Geometry: final body of the model. Coordinates: model frame, mm. A direction names the side the tool comes from. Round coordinates to 2 decimals unless told otherwise and drop trailing zeros. Write each loop counter-clockwise with the first axis right and the second up, starting at its lowest first coordinate (ties: lowest second). Pieces come first, ordered by that corner, then holes. Notation, with made-up numbers: M -14,24.25 L -3,24.25 A12 cw -3,28.25 Z; hole C 5,60 d8. An arc over 180 degrees is marked long. Answer as CSV lines item,"result". Start each with the question number.
Q1. Mould query, pull axis Y, two halves, no side actions, for faces 4 (the flat face through (12.5, -5, 2)), 5 (the cylindrical face through (1.376, 0.894, 1.504)), 6 (the conical face through (23.5, 3.3, -4.4)). Classes: pulls with the +Y half, pulls with the -Y half, needs draft (parallel to the pull), parting line crosses it, or undercut.
Q2. Reachability of faces 1 (the flat face through (5, 0, -1.75)), 2 (the flat face through (24.5, 6, -2)), 3 (the flat face through (5, 0, 1.75)) from +Z, -Z, +X, -X, +Y, -Y: full face, straight path, thin tool, end or side. Return the list, or none.
Q3. First-contact query: pin 1 (8 mm diameter, centred on x = 17, z = -3.5, fed in from -Y); pin 2 (1.3 mm diameter, centred on x = 5.5, y = -0.5, fed in from -Z); pin 3 (0.8 mm diameter, centred on x = 6, y = 0.5, fed in from +Z). Flat tips, straight axial feed; report the tip coordinate or a pass-through.
Q4. Ray query, probe 1 along Z at (x, y) = (6.25, 1); probe 2 along Z at (x, y) = (21.75, 4.5); probe 3 along Y at (x, z) = (24.25, 3.5). Return the intervals inside material, ascending.
Q5. Section query A-A on x = 6. Output: boundary loops of the cut face in (y, z), and give its area (3 significant figures).
Q6. Section query B-B on x = 10.5. Output: boundary loops of the cut face in (y, z), and give its area (3 significant figures).
```python
from build123d import *

# Parameters (mm, degrees)
CHAMFER_1_SIZE      = 0.4
FILLET_1_R          = 0.1
SKETCH_4_W          = 0.5
SKETCH_4_H          = 2.5
EXTRUDE_1_DEPTH     = 8
FILLET_2_R          = 1.25
CUT_EXTRUDE_1_DEPTH = 33.21121699


with BuildPart() as part:
    # Эскиз1 → Повернуть1 (revolve)
    with BuildSketch(Plane.XY, mode=Mode.PRIVATE) as revolve_1_sk:
        with BuildLine():
            Line((9, 0), (9, 5))
            Line((9, 5), (12.5, 5))
            Line((12.5, 5), (12.5, 6))
            Line((12.5, 6), (24.5, 6))
            Line((24.5, 6), (24.5, 9))
            Line((24.5, 9), (29, 8.206528587))
            Line((29, 8.206528587), (29, 6.869960021))
            Line((29, 6.869960021), (21.5, 5))
            ThreePointArc((21.5, 5), (25.035533906, 3.535533906), (26.5, 0))
            Line((26.5, 0), (9, 0))
        make_face()
    revolve(revolve_1_sk.sketch.rotate(Axis((9, 0, 0), (1, 0, 0)), 90), axis=Axis((9, 0, 0), (1, 0, 0)))

    # Фаска1
    chamfer_1_edges = [part.edges().sort_by_distance(p)[0] for p in [
        (12.5, 0, -6),
    ]]
    chamfer(chamfer_1_edges, length=CHAMFER_1_SIZE)

    # Скругление1
    fillet_1_edges = [part.edges().sort_by_distance(p)[0] for p in [
        (9, 0, -5),
        (29, 0, -6.869960021),
        (29, 0, -8.206528587),
    ]]
    fillet(fillet_1_edges, radius=FILLET_1_R)

    # Эскиз4 → Бобышка-Вытянуть1 (add)
    with BuildSketch(Plane.ZY.offset(-9)):
        with Locations((1.5, 0)):
            Rectangle(SKETCH_4_W, SKETCH_4_H)
        with Locations((-1.5, 0)):
            Rectangle(SKETCH_4_W, SKETCH_4_H)
    extrude(amount=EXTRUDE_1_DEPTH)

    # Скругление2
    fillet_2_edges = [part.edges().sort_by_distance(p)[0] for p in [
        (1, -1.25, 1.5),
        (1, -1.25, -1.5),
        (1, 1.25, 1.5),
        (1, 1.25, -1.5),
    ]]
    fillet(fillet_2_edges, radius=FILLET_2_R - 0.0001)  # a hair under: the kernel refuses the full size

    # Эскиз5 → Вырез-Вытянуть1 (cut, through all)
    with BuildSketch(Plane(origin=(0, 0, -1.75), x_dir=(-1, 0, 0), z_dir=(0, 0, -1))):
        with BuildLine():
            Line((-4.25, 0.5), (-2.25, 0.5))
            ThreePointArc((-2.25, 0.5), (-1.75, 0), (-2.25, -0.5))
            Line((-2.25, -0.5), (-4.25, -0.5))
            ThreePointArc((-4.25, -0.5), (-4.75, 0), (-4.25, 0.5))
        make_face()
    extrude(amount=-CUT_EXTRUDE_1_DEPTH, mode=Mode.SUBTRACT)


solid = part.part
```
Entries:
1,face 4,"needs draft"
1,face 5,"pulls with the +Y half"
1,face 6,"undercut"
2,face 1,"-Z, -X, +Y, -Y"
2,face 2,"-X"
2,face 3,"+Z, -X, +Y, -Y"
3,pin 1,"stops at y = -6"
3,pin 2,"stops at z = -1.75"
3,pin 3,"stops at z = 1.75"
4,probe 1,"z = -1.75 to -1.25, 1.25 to 1.75"
4,probe 2,"z = -3.97 to -2.32, -2.17 to 2.17, 2.32 to 3.97"
4,probe 3,"y = -4.87 to -4.48, -2.28 to 2.28, 4.48 to 4.87"
5,outline,"M -1.25,-1.75 L 1.25,-1.75 L 1.25,-1.25 L -1.25,-1.25 Z; M -1.25,1.25 L 1.25,1.25 L 1.25,1.75 L -1.25,1.75 Z"
5,area,"2.50 mm^2"
6,outline,"C 0,0 d10"
6,area,"78.5 mm^2"
